Geometry check sheet. Reference: the model listing, model coordinates, mm. A direction names the side the tool comes from. Give positions to 0.01 mm unless a question says otherwise; leave off trailing zeros. Write each loop counter-clockwise with the first axis right and the second up, starting at its lowest first coordinate (ties: lowest second). Pieces come first, ordered by that corner, then holes. Notation, with made-up numbers: (-2, -9.75) - (31, -9.75) arc R18 ccw to (31, 13.25) - close; hole circle Ø11 at (82.25, 14). An arc over 180 degrees is marked (long way). Write item = value, one per line. Start each with the question number.
(1) Thickness scan on L1, parallel to X at y = 0, z = -15; L2, parallel to X at y = -2, z = -4. Record the ranges inside material, lowest first.
(2) Draft check along X on faces 1 (the cylindrical face through (1.07, -5.95, 65.23)), 2 (the flat face through (-1, -1, -28.4)), 3 (the cylindrical face through (-53.876, -4.607, -23.302)), 4 (the cylindrical face through (53.84, -4.61, -23.38)). Enter one of: pulls with the +X half, pulls with the -X half, needs draft (parallel to the pull), parting line crosses it, or undercut.
(3) Access from +Z, -Z, +X, -X, +Y, -Y to the whole of each face (thin tool, end or side, straight path). Record for faces 5 (the flat face through (-1, -1, -25.4)), 6 (the flat face through (-5, -12.065, 59)).
(4) Depth check by flat-ended pin: pin 1 Ø6 at (x, z) = (-21.5, -16.5) entering from -Y; pin 2 Ø4 at (x, z) = (15.5, -2.5) entering from -Y; pin 3 Ø1 at (x, z) = (53.5, -24.5) entering from -Y. Enter the tip coordinate at first touch or a pass-through.
(5) Section check C-C, the plane z = -16. Enter the section's corners in (x, y), plus the area to 3 significant figures.
(6) Section check A-A, the plane z = 52.5. Enter the section's corners in (x, y) (3 decimals), plus the area to 3 significant figures.
(7) Section check B-B, the plane x = 0. Enter the section's corners in (y, z) (3 decimals), plus the area to 3 significant figures.
```python
from build123d import *

# Parameters (mm, degrees)
F0_R          = 65.2372499689
F0_R_2        = 58.6990889692
F1_DEPTH      = 12.065
F2_R          = 66.0831305436
F2_R_2        = 55.1753254818
F3_DEPTH      = 25.4
F3_TAPER      = -3
F3_DEPTH_BACK = 25.4
F5_DEPTH      = 50.25
F6_R          = 66.0831305436
F7_DEPTH      = 3


with BuildPart() as f1:
    # F0 (on Front) → F1 (new body)
    with BuildSketch(Plane.XZ):
        Circle(F0_R)
        Circle(F0_R_2, mode=Mode.SUBTRACT)
    extrude(amount=F1_DEPTH)

    # F2 (on Top) → F3 (join, two sides)
    with BuildSketch(Plane.XY) as f3_sk:
        Circle(F2_R)
        Circle(F2_R_2, mode=Mode.SUBTRACT)
    extrude(amount=F3_DEPTH, taper=F3_TAPER)
    extrude(f3_sk.sketch, amount=-F3_DEPTH_BACK)

    # F4 (on Front) → F5 (cut)
    with BuildSketch(Plane.XZ):
        Polygon((66.0831305436, -25.4), (-66.0831305436, -25.4), (-61.7706626654, -79.2663544416), (70.8459764719, -79.2663544416), align=None)
    extrude(amount=F5_DEPTH, mode=Mode.SUBTRACT)

    # F6 (on face) → F7 (join)
    with BuildSketch(Plane(origin=(0, 0, -25.4), x_dir=(1, 0, 0), z_dir=(0, 0, -1))):
        Circle(F6_R)
    extrude(amount=F7_DEPTH)


solid = f1.part
```
Model answer:
q1.L1 = -66.08 to -55.18, 55.18 to 66.08
q1.L2 = -66.05 to -55.14, 55.14 to 66.05
q2.face_1 = parting line crosses it
q2.face_2 = needs draft
q2.face_3 = undercut
q2.face_4 = undercut
q3.face_5 = none
q3.face_6 = +Z, +X, -X, -Y
q4.pin_1 = -63.44
q4.pin_2 = -64.69
q4.pin_3 = -39.47
q5.outline = circle Ø132.17 at (0, 0); hole circle Ø110.35 at (0, 0)
q5.area = 4,160 mm²
q6.outline = (-38.725, -12.065) - (-26.255, -12.065) - (-26.255, 0) - (-38.725, 0) - close; (26.255, -12.065) - (38.725, -12.065) - (38.725, 0) - (26.255, 0) - close
q6.area = 301 mm²
q7.outline = (-67.414, 25.4) - (-66.083, 0) - (-66.083, -28.4) - (66.083, -28.4) - (66.083, 0) - (67.414, 25.4) - (53.844, 25.4) - (55.175, 0) - (55.175, -25.4) - (-55.175, -25.4) - (-55.175, 0) - (-53.844, 25.4) - close; (-12.065, 58.699) - (0, 58.699) - (0, 65.237) - (-12.065, 65.237) - close
q7.area = 1,650 mm²
